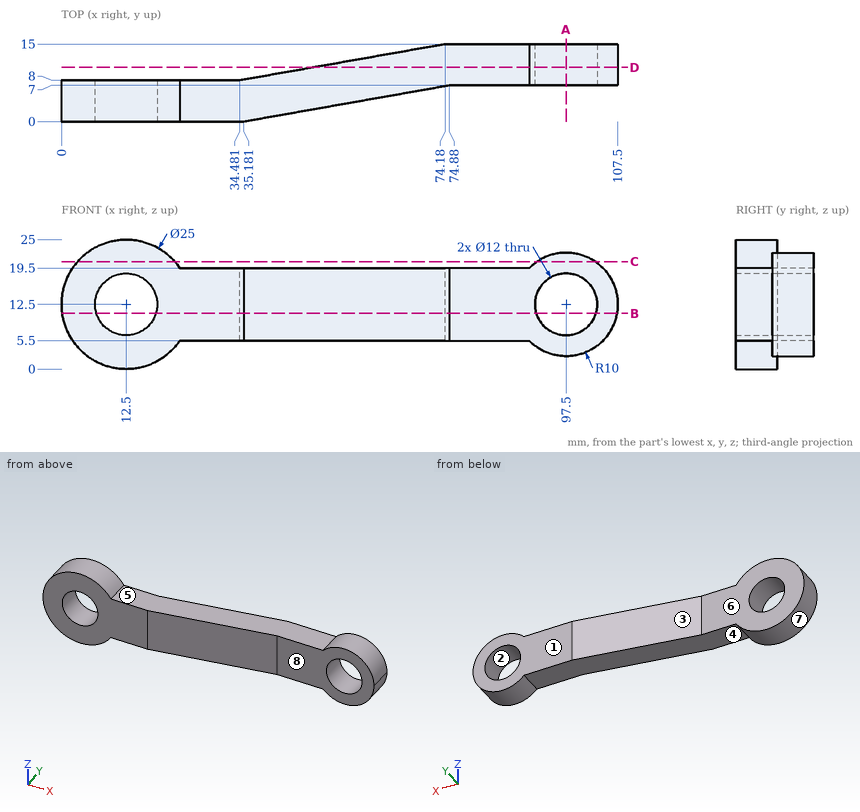
Input: dimensioned drawing with shaded views. Units: mm. Origin: part minimum x, y, z. A direction names the side the tool comes from. Coordinates: 2 decimals unless noted, no trailing zeros. Order: outer loops, then holes, each group sorted by start corner. A loop starts at its lowest first (then second) coordinate and runs counter-clockwise, first axis right, second up. Notation, with made-up numbers: (73.25, -38.5) -> (81.25, -38.5) arc R9 ccw to (81.25, -33.5) -> close; hole circle Ø6 at (-3.75, 50). An arc over 180 degrees is marked (long way). Use CSV: the item, a comma, the result in double quotes.
1) Section B-B on z = 10.75. Output: boundary loops of the cut face in (x, y).
Findings:
outline,"(0.12, 0) -> (6.76, 0) -> (6.76, 8) -> (0.12, 8) -> close; (18.24, 0) -> (35.18, 0) -> (74.88, 7) -> (91.76, 7) -> (91.76, 15) -> (74.18, 15) -> (34.48, 8) -> (18.24, 8) -> close; (103.24, 7) -> (107.35, 7) -> (107.35, 15) -> (103.24, 15) -> close"
2) Section C-C on z = 20.75. Output: boundary loops of the cut face in (x, y), then the cut area to 3 significant figures.
Findings:
outline,"(3.11, 0) -> (21.89, 0) -> (21.89, 8) -> (3.11, 8) -> close; (91.85, 7) -> (103.15, 7) -> (103.15, 15) -> (91.85, 15) -> close"
area,"241 mm^2"
3) Access query for the marked faces 4, 5, 6, 7 and 8. Directions: +Z, -Z, +X, -X, +Y, -Y. A direction counts if a zero-diameter tool reaches every point of the face in a straight line with its end or side. Return the directions, or none.
Findings:
face 4,"-Z, +Y, -Y"
face 5,"+Z, +Y, -Y"
face 6,"+Z, -Z, -X, +Y"
face 7,"+Y, -Y"
face 8,"+Z, -Z, +X, -Y"
4) Pin query (flat end, axial travel): pin 1 Ø4 at (x, y) = (81.5, 11.5) entering from +Z; pin 2 Ø5 at (x, z) = (57, 15) entering from +Y; pin 3 Ø1 at (y, z) = (2.5, 22) entering from +X (1 decimal). Return the tip coordinate at first contact, or that it passes through.
Findings:
pin 1,"stops at z = 19.5"
pin 2,"stops at y = 12.41"
pin 3,"stops at x = 21.2"
5) Section D-D on y = 10.5. Output: boundary loops of the cut face in (x, z), then the cut area to 3 significant figures.
Findings:
outline,"(48.66, 5.5) -> (90.36, 5.5) arc R10 ccw (long way) to (90.36, 19.5) -> (48.66, 19.5) -> close; hole circle Ø12 at (97.5, 12.5)"
area,"757 mm^2"
6) Section A-A on x = 97.5. Output: boundary loops of the cut face in (y, z), then the cut area to 3 significant figures.
Findings:
outline,"(7, 2.5) -> (15, 2.5) -> (15, 6.5) -> (7, 6.5) -> close; (7, 18.5) -> (15, 18.5) -> (15, 22.5) -> (7, 22.5) -> close"
area,"64.0 mm^2"
7) Mould query, pull axis X, two halves, no side actions, for the marked faces 1, 2 and 3. Classes: +X half, -X half, draft (parallel to the pull), parting line (faces both ways), or undercut.
Findings:
face 1,"draft"
face 2,"undercut"
face 3,"-X half"
8) Line query: line 1 (Z direction, x = 97.5, y = 13); line 2 (Z direction, x = 12.5, y = 1.75); line 3 (Y direction, x = 75, z = 6.5). Output: solid intervals per line, ascending.
Findings:
line 1,"z = 2.5 to 6.5, 18.5 to 22.5"
line 2,"z = 0 to 6.5, 18.5 to 25"
line 3,"y = 7 to 15"
